The figure shows three views and two pictorial views of one solid part (mm, origin at its lowest corner). Answer the questions. Give positions to 0.01 mm unless a question says otherwise; leave off trailing zeros. Loops run counter-clockwise (first coordinate to the right, second up) from the corner with the lowest first, then second, coordinate; pieces in that order, holes last. Notation, with made-up numbers: (12.25, 18) -> (40.25, 18) arc R19 ccw to (40.25, 52) -> close; hole circle Ø6 at (33.5, 0). An arc over 180 degrees is marked (long way). Answer as CSV lines item,"result". Start each with the question number.
1. Find section C-C, the plane y = 0.6. Count the separate pieces of the cut face and the enclosed holes in it, and give its area (3 significant figures).
2. Find section A-A, the plane x = 134.62. Give the vertices of the cut face in (y, z) (1 decimal).
3. Find the intervals of material crossed by line 1 along Z through (x, y) = (161, 0.4) (1 decimal); line 2 along Z through (x, y) = (12.5, 1.1); line 3 along Y through (x, z) = (158, 51), in increasing order.
4. Find section B-B, the plane z = 54.61. Give the vertices of the cut face in (x, y) (1 decimal).
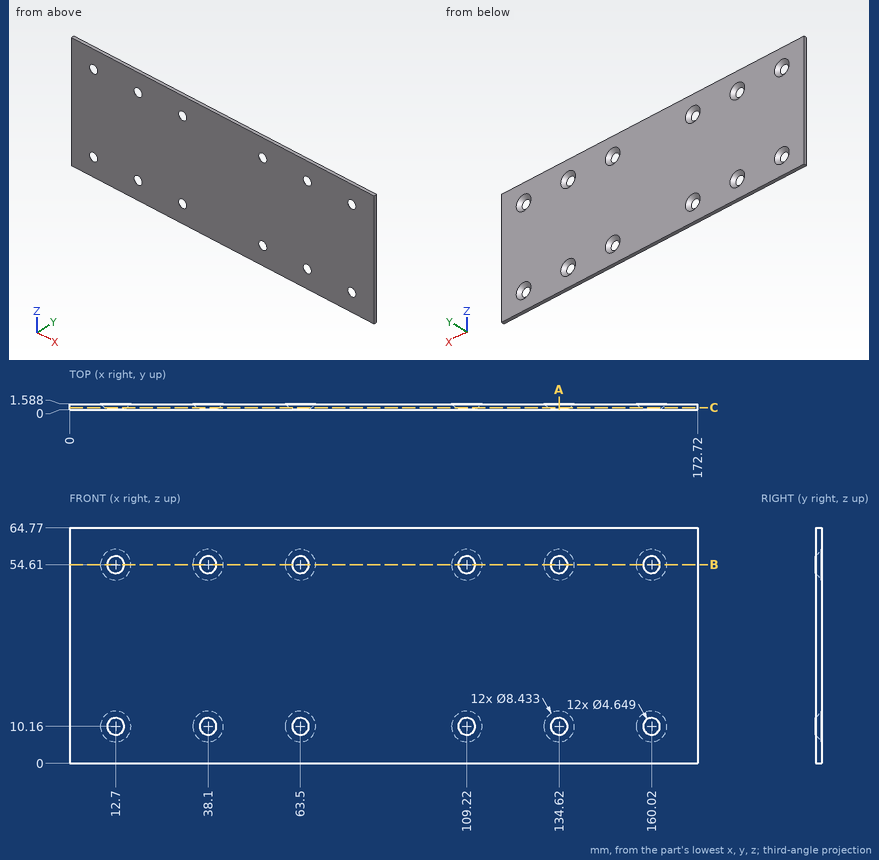
Resolved:
1,separate pieces,"1"
1,enclosed holes,"12"
1,area,"10,800 mm^2"
2,outline,"(0, 0) -> (1.6, 0) -> (1.6, 5.9) -> (0, 7.8) -> close; (0, 12.5) -> (1.6, 14.4) -> (1.6, 50.4) -> (0, 52.3) -> close; (0, 56.9) -> (1.6, 58.8) -> (1.6, 64.8) -> (0, 64.8) -> close"
3,line 1,"z = 0 to 7.5, 12.8 to 52, 57.2 to 64.8"
3,line 2,"z = 0 to 6.53, 13.79 to 50.98, 58.24 to 64.77"
3,line 3,"y = 0 to 1.52"
4,outline,"(0, 0) -> (10.4, 0) -> (8.5, 1.6) -> (0, 1.6) -> close; (15, 0) -> (35.8, 0) -> (33.9, 1.6) -> (16.9, 1.6) -> close; (40.4, 0) -> (61.2, 0) -> (59.3, 1.6) -> (42.3, 1.6) -> close; (65.8, 0) -> (106.9, 0) -> (105, 1.6) -> (67.7, 1.6) -> close; (111.5, 0) -> (132.3, 0) -> (130.4, 1.6) -> (113.4, 1.6) -> close; (136.9, 0) -> (157.7, 0) -> (155.8, 1.6) -> (138.8, 1.6) -> close; (162.3, 0) -> (172.7, 0) -> (172.7, 1.6) -> (164.2, 1.6) -> close"
